from build123d import *

# Parameters (mm, degrees)
SKETCH2_W           = 52
SKETCH2_H           = 120
SKETCH2_R           = 1.75
BOSS_EXTRUDE1_DEPTH = 5
CUT_EXTRUDE1_DEPTH  = 6
SKETCH4_R           = 4.55
BOSS_EXTRUDE2_DEPTH = 15
SKETCH5_W           = 2
SKETCH5_H           = 2.611250176
CUT_EXTRUDE2_DEPTH  = 121
FILLET1_R           = 5


with BuildPart() as part:
    # Sketch2 → Boss-Extrude1 (new body)
    with BuildSketch(Plane(origin=(0, 0, 0), x_dir=(1, 0, 0), z_dir=(0, 1, 0))):
        with Locations((26, 60)):
            Rectangle(SKETCH2_W, SKETCH2_H)
        with Locations((6, 7.5)):
            Circle(SKETCH2_R, mode=Mode.SUBTRACT)
        with Locations((46, 7.5)):
            Circle(SKETCH2_R, mode=Mode.SUBTRACT)
        with Locations((6, 112.5)):
            Circle(SKETCH2_R, mode=Mode.SUBTRACT)
        with Locations((46, 112.5)):
            Circle(SKETCH2_R, mode=Mode.SUBTRACT)
    extrude(amount=BOSS_EXTRUDE1_DEPTH)

    # Sketch3 → Cut-Extrude1 (cut, through all)
    with BuildSketch(Plane(origin=(0, 5, 0), x_dir=(1, 0, 0), z_dir=(0, 1, 0))):
        Polygon((0, 105), (16, 85), (16, 35), (0, 15), align=None)
        Polygon((52, 105), (36, 85), (36, 35), (52, 15), align=None)
    extrude(amount=-CUT_EXTRUDE1_DEPTH, mode=Mode.SUBTRACT)

    # Sketch4 → Boss-Extrude2 (add)
    with BuildSketch(Plane(origin=(0, 0, -120), x_dir=(-1, 0, 0), z_dir=(0, 0, -1))):
        with BuildLine():
            Line((-33.05, 12.05), (-33.05, 5))
            Line((-33.05, 5), (-18.95, 5))
            Line((-18.95, 5), (-18.95, 12.05))
            ThreePointArc((-18.95, 12.05), (-26, 19.1), (-33.05, 12.05))
        make_face()
        with Locations((-26, 12.05)):
            Circle(SKETCH4_R, mode=Mode.SUBTRACT)
    extrude(amount=-BOSS_EXTRUDE2_DEPTH)

    # Sketch5 → Cut-Extrude2 (cut, through all)
    with BuildSketch(Plane(origin=(0, 0, -120), x_dir=(-1, 0, 0), z_dir=(0, 0, -1))):
        with Locations((-26, 17.794374912)):
            Rectangle(SKETCH5_W, SKETCH5_H)
    extrude(amount=-CUT_EXTRUDE2_DEPTH, mode=Mode.SUBTRACT)

    # Fillet1
    fillet1_edges = [part.edges().sort_by_distance(p)[0] for p in [
        (0, 2.5, -15),
        (0, 2.5, -105),
        (16, 2.5, -85),
        (16, 2.5, -35),
        (52, 2.5, -105),
        (52, 2.5, -15),
        (36, 2.5, -35),
        (36, 2.5, -85),
        (18.95, 5, -112.5),
        (33.05, 5, -112.5),
        (0, 2.5, -120),
        (52, 2.5, -120),
        (52, 2.5, 0),
        (0, 2.5, 0),
    ]]
    fillet(fillet1_edges, radius=FILLET1_R)


solid = part.part
Could you check a few things on this model? Use its own coordinates, in mm. A direction names the side the tool comes from. Give positions to 0.01 mm unless a question says otherwise; leave off trailing zeros. Write each loop counter-clockwise with the first axis right and the second up, starting at its lowest first coordinate (ties: lowest second). Pieces come first, ordered by that corner, then holes. Notation, with made-up numbers: (-32.75, 36) - (9.25, 36) arc R27 ccw to (9.25, 59) - close; hole circle Ø6 at (-32.75, 75). An arc over 180 degrees is marked (long way). Use CSV: the item, a comma, the result in double quotes. Start each with the question number.
Item 1: I want a section at B-B, the plane z = -99. Please give me the cut outline in (x, y).
Item 2: I'm going to push flat-ended pins straight in: pin 1 (4.5 mm diameter, centred on x = 6, z = -112.5, fed in from +Y); pin 2 (7.5 mm diameter, centred on x = 26, y = 12.05, fed in from +Z); pin 3 (1.5 mm diameter, centred on y = 1.5, z = -67.5, fed in from +X); pin 4 (0.6 mm diameter, centred on y = 10.5, z = -114, fed in from -X). Where does each tip first touch, or does it pass through?
Item 3: For faces 1 (the face through (5.772, 2.465, -114.235)), 2 (the face through (27, 7, -105)), 3 (the face through (15.71, 2.46, -84.92)), 4 (the face through (36.274, 2.465, -84.879)), 5 (the face through (33.05, 11, -113)), which set-ups out of +Z, -Z, +X, -X, +Y, -Y let a thin tool reach every point of the face, with its end or its side?
Item 4: I want a section at C-C, the plane z = -56.5. Please give me the cut outline in (x, y), then the cut area to 3 significant figures.
Item 5: I want a section at A-A, the plane z = -112.5. Please give me the cut outline in (x, y).
Item 6: If we mould it in two halves opening along Z, with no side actions, what happens to faces 6 (the face through (17.52, 6.5, -112.4)), 7 (the face through (0.274, 2.465, -14.879)), 8 (the face through (26, 5, -120)), 9 (the face through (16, 3, -60))? For each: pulls with the +Z half, pulls with the -Z half, needs draft (parallel to the pull), parting line crosses it, or undercut.
Item 7: If I drill on line 1 along X through (y, z) = (3.5, -112.5); line 2 along Z through (x, y) = (6, 1.75); line 3 along Y through (x, z) = (26.5, -45.5), over which ranges is the centre line in solid material (lowest first)?
Findings:
1,outline,"(4.8, 0) - (47.2, 0) - (47.2, 5) - (4.8, 5) - close"
2,pin 1,"stops at y = 5"
2,pin 2,"passes through"
2,pin 3,"stops at x = 36"
2,pin 4,"stops at x = 18.95"
3,face 1,"+Y, -Y"
3,face 2,"+Z, +X, -X, +Y"
3,face 3,"-X, +Y, -Y"
3,face 4,"+X, +Y, -Y"
3,face 5,"+Z, -Z, +X, +Y"
4,outline,"(16, 0) - (36, 0) - (36, 5) - (16, 5) - close"
4,area,"100 mm2"
5,outline,"(0, 0) - (4.25, 0) - (4.25, 5) - (0, 5) - close; (7.75, 0) - (44.25, 0) - (44.25, 5) - (38.05, 5) arc R5 cw to (33.05, 10) - (33.05, 12.05) arc R7.05 ccw to (27, 19.03) - (27, 16.49) arc R4.55 cw (long way) to (25, 16.49) - (25, 19.03) arc R7.05 ccw to (18.95, 12.05) - (18.95, 10) arc R5 cw to (13.95, 5) - (7.75, 5) - close; (47.75, 0) - (52, 0) - (52, 5) - (47.75, 5) - close"
6,face 6,"needs draft"
6,face 7,"undercut"
6,face 8,"pulls with the -Z half"
6,face 9,"undercut"
7,line 1,"x = 0 to 4.25, 7.75 to 44.25, 47.75 to 52"
7,line 2,"z = -120 to -114.25, -110.75 to -97.5, -22.5 to -9.25, -5.75 to 0"
7,line 3,"y = 0 to 5"
